The listing builds one solid part. Answer for the finished solid, in the listing's coordinates (mm). A direction names the side the tool comes from. Round coordinates to 2 decimals unless told otherwise and drop trailing zeros. Loops run counter-clockwise (first coordinate to the right, second up) from the corner with the lowest first, then second, coordinate; pieces in that order, holes last. Notation, with made-up numbers: (-34, 23) - (22, 23) arc R10 ccw to (22, 38) - close; hole circle Ø8 at (5, 30.25). An arc over 180 degrees is marked (long way). One line per question, with ' | ' between items. Start each with the question number.
from build123d import *

# Parameters (mm, degrees)
F0_W     = 50.8
F0_H     = 50.8
F0_R     = 6.35
F2_DEPTH = 12.7
F1_W     = 50.8
F1_H     = 50.8
F3_DEPTH = 12.7


with BuildPart() as f2:
    # F0 (on Front) → F2 (new body)
    with BuildSketch(Plane.XZ):
        with Locations((25.4, 25.4)):
            Rectangle(F0_W, F0_H)
        with Locations((26.411066, 26.928931)):
            Circle(F0_R, mode=Mode.SUBTRACT)
    extrude(amount=F2_DEPTH)

    # F1 (on Top) → F3 (join)
    with BuildSketch(Plane.XY):
        with Locations((25.4, 25.4)):
            Rectangle(F1_W, F1_H)
    extrude(amount=F3_DEPTH)


solid = f2.part
(1) Find section D-D on x = 18.5. Write down the section's boundary in (y, z).
(2) Find section C-C on y = 45. Write down the section's boundary in (x, z), plus the area to 3 significant figures.
(3) Find section B-B on z = 31.5. Write down the section's boundary in (x, y).
(4) A tool of negligible diameter and unlimited length cuts with its end or side. For faces 1 (the flat face through (25, 0, 36)), 2 (the flat face through (50.8, 4, 8)), from which of +Z, -Z, +X, -X, +Y, -Y can it reach the whole face along a straight path? Write none if from no direction.
(5) Consider L1, parallel to Z at x = 12, y = 41; L2, parallel to Y at x = 46, z = 48; L3, parallel to Z at x = 32, y = -1. Determine where each line is inside the solid, lowest interval first.
(6) Each of these flat-tipped pins is pushed along its axis until it touches: P1, Ø12, axis at x = 34.5, z = 26.5, coming from the +Y side; P2, Ø12, axis at x = 27.5, y = 43, coming from the +Z side. Where does it stop, or does it pass through?
(7) Determine the mould class of faces 3 (the flat face through (25, 26, 12.7)), 4 (the flat face through (0, 4, 8)), 5 (the cylindrical face through (32.28, -6.26, 24.5)) for opening direction Z: pulls with the +Z half, pulls with the -Z half, needs draft (parallel to the pull), parting line crosses it, or undercut.
(8) Find section A-A on x = 31. Write down the section's boundary in (y, z), plus the area to 3 significant figures.
Answer below:
1) outline: (-12.7, 0) - (50.8, 0) - (50.8, 12.7) - (0, 12.7) - (0, 50.8) - (-12.7, 50.8) - close
2) outline: (0, 0) - (50.8, 0) - (50.8, 12.7) - (0, 12.7) - close | area: 645 mm2
3) outline: (0, -12.7) - (22, -12.7) - (22, 0) - (0, 0) - close; (30.82, -12.7) - (50.8, -12.7) - (50.8, 0) - (30.82, 0) - close
4) face 1: +Z, +X, -X, +Y | face 2: +Z, -Z, +X, +Y, -Y
5) L1: 0 to 12.7 | L2: -12.7 to 0 | L3: 0 to 23.91, 29.94 to 50.8
6) P1: y = 0 | P2: z = 12.7
7) face 3: pulls with the +Z half | face 4: needs draft | face 5: undercut
8) outline: (-12.7, 0) - (50.8, 0) - (50.8, 12.7) - (0, 12.7) - (0, 22.54) - (-12.7, 22.54) - close; (-12.7, 31.32) - (0, 31.32) - (0, 50.8) - (-12.7, 50.8) - close | area: 1,180 mm2
